Geometry: final body of the model. Coordinates: model frame, mm. A direction names the side the tool comes from. Coordinates: 2 decimals unless noted, no trailing zeros. Order: outer loops, then holes, each group sorted by start corner. A loop starts at its lowest first (then second) coordinate and runs counter-clockwise, first axis right, second up. Notation, with made-up numbers: (-36, -3.5) - (15, -3.5) arc R20 cw to (15, 25.5) - close; hole circle Ø10 at (39.5, 44.5). An arc over 180 degrees is marked (long way). Use a Markdown table: item, result. Add a question column.
```python
from build123d import *

# Parameters (mm, degrees)
F0_W     = 25
F0_H     = 2
F0_W_2   = 7.75
F0_H_2   = 34.2
F1_DEPTH = 30
F0_W_3   = 12.5
F2_DEPTH = 2.4
F3_R     = 5


with BuildPart() as f1:
    # F0 (on Top) → F1 (new body)
    with BuildSketch(Plane.XY):
        Polygon((-90.5, -19.1), (-70.25, -19.1), (-70.25, -17.1), (-82.75, -17.1), (-82.75, 17.1), (-70.25, 17.1), (-70.25, 19.1), (-90.5, 19.1), align=None)
        with Locations((-57.75, -18.1)):
            Rectangle(F0_W, F0_H)
        Polygon((-45.25, -19.1), (-12.5, -19.1), (-12.5, -17.1), (-25, -17.1), (-32.75, -17.1), (-45.25, -17.1), align=None)
        Polygon((-12.5, 17.1), (-12.5, 19.1), (-45.25, 19.1), (-45.25, 17.1), (-32.75, 17.1), (-25, 17.1), align=None)
        with Locations((0, -18.1)):
            Rectangle(F0_W, F0_H)
        Polygon((12.5, -19.1), (45.25, -19.1), (45.25, -17.1), (32.75, -17.1), (25, -17.1), (12.5, -17.1), align=None)
        with Locations((57.75, -18.1)):
            Rectangle(F0_W, F0_H)
        Polygon((70.25, -19.1), (90.5, -19.1), (90.5, 19.1), (70.25, 19.1), (70.25, 17.1), (82.75, 17.1), (82.75, -17.1), (70.25, -17.1), align=None)
        Polygon((45.25, 17.1), (45.25, 19.1), (12.5, 19.1), (12.5, 17.1), (25, 17.1), (32.75, 17.1), align=None)
        with Locations((28.875, 0)):
            Rectangle(F0_W_2, F0_H_2)
        with Locations((-28.875, 0)):
            Rectangle(F0_W_2, F0_H_2)
    extrude(amount=F1_DEPTH)

    # F0 (on Top) → F2 (join)
    with BuildSketch(Plane.XY):
        with Locations((-57.75, 18.1)):
            Rectangle(F0_W, F0_H)
        with Locations((-76.5, 0)):
            Rectangle(F0_W_3, F0_H_2)
        with Locations((-57.75, 0)):
            Rectangle(F0_W, F0_H_2)
        with Locations((-39, 0)):
            Rectangle(F0_W_3, F0_H_2)
        with Locations((-18.75, 0)):
            Rectangle(F0_W_3, F0_H_2)
        Rectangle(F0_W, F0_H_2)
        with Locations((0, 18.1)):
            Rectangle(F0_W, F0_H)
        with Locations((18.75, 0)):
            Rectangle(F0_W_3, F0_H_2)
        with Locations((39, 0)):
            Rectangle(F0_W_3, F0_H_2)
        with Locations((57.75, 0)):
            Rectangle(F0_W, F0_H_2)
        with Locations((57.75, 18.1)):
            Rectangle(F0_W, F0_H)
        with Locations((76.5, 0)):
            Rectangle(F0_W_3, F0_H_2)
    extrude(amount=F2_DEPTH)

    # F3
    f3_edges = [f1.edges().sort_by_distance(p)[0] for p in [
        (-70.25, 18.1, 30),
        (-45.25, 18.1, 30),
        (-12.5, 18.1, 30),
        (12.5, 18.1, 30),
        (45.25, 18.1, 30),
        (70.25, 18.1, 30),
    ]]
    fillet(f3_edges, radius=F3_R)


solid = f1.part
```
1) Section query C-C (y = -12). Return the cut outline in (x, z), and give its area (3 significant figures).
2) Section query D-D (x = 67). Return the cut outline in (y, z).
3) Access query for faces 3 (the cylindrical face through (-43.82, 18.09, 28.5)), 4 (the flat face through (-39, 17.1, 16)), 5 (the flat face through (90.5, 0, 15)). Directions: +Z, -Z, +X, -X, +Y, -Y. A direction counts if a zero-diameter tool reaches every point of the face in a straight line with its end or side. Return the directions, or none.
4) First-contact query: pin 1 (5 mm diameter, centred on x = -51, y = -11, fed in from -Z); pin 2 (8.5 mm diameter, centred on x = 58.5, z = 23, fed in from +Y); pin 3 (18 mm diameter, centred on x = 10.5, y = -1, fed in from +Z). Flat tips, straight axial feed; report the tip coordinate or a pass-through.
5) Section query B-B (x = 19.5). Return the cut outline in (y, z), and give its area (3 significant figures).
6) Section query A-A (z = 9.25). Return the cut outline in (x, y).
7) Line query: line 1 (X direction, y = -9, z = 20.75); line 2 (Y direction, x = -19.5, z = 16.5); line 3 (Z direction, x = 50, y = -13). Output: solid intervals per line, ascending. Write a range as from..to.
8) Draft query along Y for faces 1 (the cylindrical face through (43.82, 18.11, 28.5)), 2 (the flat face through (-19, 17.1, 16)). Return one class per face: released by +Y, released by -Y, zero draft, split by the parting line, or undercut.
From the geometry:
| question | item | result |
|---|---|---|
| 1 | outline | (-90.5, 0) - (90.5, 0) - (90.5, 30) - (82.75, 30) - (82.75, 2.4) - (32.75, 2.4) - (32.75, 30) - (25, 30) - (25, 2.4) - (-25, 2.4) - (-25, 30) - (-32.75, 30) - (-32.75, 2.4) - (-82.75, 2.4) - (-82.75, 30) - (-90.5, 30) - close |
| 1 | area | 1,290 mm^2 |
| 2 | outline | (-19.1, 0) - (19.1, 0) - (19.1, 2.4) - (-17.1, 2.4) - (-17.1, 30) - (-19.1, 30) - close |
| 3 | face 3 | +Z, +Y |
| 3 | face 4 | +Z |
| 3 | face 5 | +Z, -Z, +X, +Y, -Y |
| 4 | pin 1 | stops at z = 0 |
| 4 | pin 2 | stops at y = -17.1 |
| 4 | pin 3 | stops at z = 2.4 |
| 5 | outline | (-19.1, 0) - (19.1, 0) - (19.1, 30) - (17.1, 30) - (17.1, 2.4) - (-17.1, 2.4) - (-17.1, 30) - (-19.1, 30) - close |
| 5 | area | 202 mm^2 |
| 6 | outline | (-90.5, -19.1) - (90.5, -19.1) - (90.5, 19.1) - (70.25, 19.1) - (70.25, 17.1) - (82.75, 17.1) - (82.75, -17.1) - (32.75, -17.1) - (32.75, 17.1) - (45.25, 17.1) - (45.25, 19.1) - (12.5, 19.1) - (12.5, 17.1) - (25, 17.1) - (25, -17.1) - (-25, -17.1) - (-25, 17.1) - (-12.5, 17.1) - (-12.5, 19.1) - (-45.25, 19.1) - (-45.25, 17.1) - (-32.75, 17.1) - (-32.75, -17.1) - (-82.75, -17.1) - (-82.75, 17.1) - (-70.25, 17.1) - (-70.25, 19.1) - (-90.5, 19.1) - close |
| 7 | line 1 | x = -90.5..-82.75, -32.75..-25, 25..32.75, 82.75..90.5 |
| 7 | line 2 | y = -19.1..-17.1, 17.1..19.1 |
| 7 | line 3 | z = 0..2.4 |
| 8 | face 1 | zero draft |
| 8 | face 2 | undercut |
